Build history of the part. All positions in model axes, mm. Face numbers are marked on the shaded views. A direction names the side the tool comes from. Give positions to 0.01 mm unless a question says otherwise; leave off trailing zeros. Order: outer loops, then holes, each group sorted by start corner. A loop starts at its lowest first (then second) coordinate and runs counter-clockwise, first axis right, second up. Notation, with made-up numbers: M 19.5,-30 L 31.5,-30 A32 ccw 31.5,0 Z; hole C 28,-26.75 d4. An arc over 180 degrees is marked long. Use CSV: the item, a comma, the result in double quotes. Start each with the question number.
Item 1: Pin check, flat tips, straight feed: P1, Ø23, axis at y = 56.5, z = 5.5, coming from the -X side; P2, Ø8, axis at x = -47, y = 129.5, coming from the +Z side; P3, Ø5, axis at x = -27, y = 197.5, coming from the -Z side. Stop position of each tip, or through.
Item 2: Which spindle directions (+Z, -Z, +X, -X, +Y, -Y) get a long thin tool onto all of the face, cutting with end or side? Do the marked faces 4, 5 and 6. Say none if no direction does.
Item 3: Band-saw the part on B-B on x = 0. Write the cut outline in (y, z), plus the area to 3 significant figures.
Item 4: Band-saw the part on A-A on z = 0. Write the cut outline in (x, y), plus the area to 3 significant figures.
Item 5: Band-saw the part on C-C on x = -40. Write the cut outline in (y, z).
Item 6: Two-plate mould, pull along Y, no slides. Class the marked faces 1, 2 and 3: pulls with the +Y half, pulls with the -Y half, needs draft (parallel to the pull), parting line crosses it, or undercut.
Item 7: Band-saw the part on D-D on y = 165. Write the cut outline in (x, z), plus the area to 3 significant figures.
Item 8: Wall check: line 1 along Y through (x, z) = (-44.5, 4.5); line 2 along Y through (x, z) = (-59.5, 35); line 3 along X through (y, z) = (125, 28). Give the ranges that are in metal, low to high.
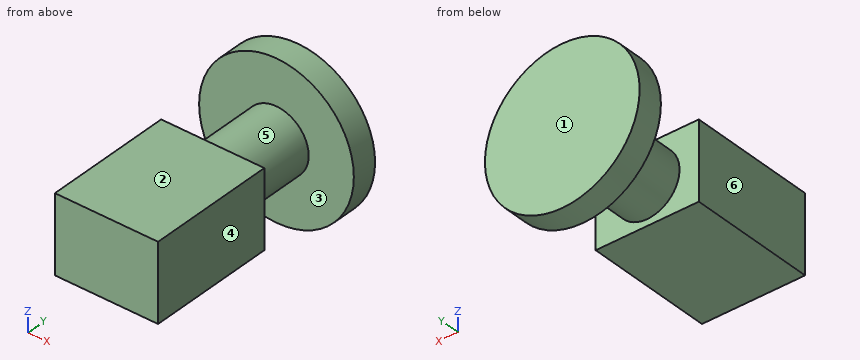
Autodesk Inventor part; units mm, degrees
ref_plane "YZ Plane" through (0, 0, 0) normal (1, 0, 0) x (0, 1, 0)
ref_plane "XZ Plane" through (0, 0, 0) normal (0, 1, 0) x (-1, 0, 0)
ref_plane "XY Plane" through (0, 0, 0) normal (0, 0, 1) x (1, 0, 0)
sketch "Sketch1" plane through (0, 0, 0) normal (0, 1, 0) x (-1, 0, 0)
  line L0 (-50.8, -38.1) -> (50.8, -38.1)
  line L1 (50.8, -38.1) -> (50.8, 38.1)
  line L2 (50.8, 38.1) -> (-50.8, 38.1)
  line L3 (-50.8, 38.1) -> (-50.8, -38.1)
  line L4 (-50.8, -38.1) -> (50.8, 38.1) construction
  line L5 (50.8, -38.1) -> (-50.8, 38.1) construction
  point P0 (0, 0)
  dimension "d0" = 101.6
  dimension "d1" = 76.2
extrude "Extrusion1" add sketch "Sketch1" along normal blind 127
sketch "Sketch2" plane through (0, 127, 0) normal (0, 1, 0) x (1, 0, 0)
  circle A0 centre (0, 0) radius 31.75
  dimension "d4" = 63.5
extrude "Extrusion2" add sketch "Sketch2" along normal blind 76.2
sketch "Sketch3" plane through (0, 203.2, 0) normal (0, 1, 0) x (1, 0, 0)
  circle A0 centre (0, 0) radius 76.2
  dimension "d7" = 152.4
extrude "Extrusion3" add sketch "Sketch3" along normal blind 25.4
properties part number "medidorPresion" material "Thermoplastic Resin"
Model answer:
1,P1,"stops at x = -50.8"
1,P2,"stops at z = 38.1"
1,P3,"stops at z = -20.19"
2,face 4,"+Z, -Z, +X, -Y"
2,face 5,"none"
2,face 6,"+Z, -Z, -X, -Y"
3,outline,"M 0,-38.1 L 127,-38.1 L 127,-31.75 L 203.2,-31.75 L 203.2,-76.2 L 228.6,-76.2 L 228.6,76.2 L 203.2,76.2 L 203.2,31.75 L 127,31.75 L 127,38.1 L 0,38.1 Z"
3,area,"18,400 mm^2"
4,outline,"M -76.2,203.2 L -31.75,203.2 L -31.75,127 L -50.8,127 L -50.8,0 L 50.8,0 L 50.8,127 L 31.75,127 L 31.75,203.2 L 76.2,203.2 L 76.2,228.6 L -76.2,228.6 Z"
4,area,"21,600 mm^2"
5,outline,"M 0,-38.1 L 127,-38.1 L 127,38.1 L 0,38.1 Z; M 203.2,-64.86 L 228.6,-64.86 L 228.6,64.86 L 203.2,64.86 Z"
6,face 1,"pulls with the +Y half"
6,face 2,"needs draft"
6,face 3,"undercut"
7,outline,"C 0,0 d63.5"
7,area,"3,170 mm^2"
8,line 1,"y = 0 to 127, 203.2 to 228.6"
8,line 2,"y = 203.2 to 228.6"
8,line 3,"x = -50.8 to 50.8"
